Read the model definition and answer for the solid it produces. Units are mm, in the model's axes. Face numbers are marked on the shaded views. Coordinates: 2 decimals unless noted, no trailing zeros. Order: outer loops, then holes, each group sorted by start corner. A loop starts at its lowest first (then second) coordinate and runs counter-clockwise, first axis right, second up. Notation, with made-up numbers: (49, 62.25) - (104, 62.25) arc R23 cw to (104, 72.25) - close; hole circle Ø4 at (64, 36). An arc over 180 degrees is marked (long way). Write item = value, one per line.
from build123d import *

# Parameters (mm, degrees)
F1_DEPTH = 6.6802
F2_DEPTH = 3.2512
F4_DEPTH = 2.54


with BuildPart() as f1:
    # F0 (on Top) → F1 (new body)
    with BuildSketch(Plane.XY):
        Polygon((46.99, 18.161), (-46.99, 18.161), (-46.99, 4.401166), (-10.16, 4.401166), (10.16, 4.401166), (46.99, 4.401166), align=None)
    extrude(amount=F1_DEPTH)

    # F0 (on Top) → F2 (join)
    with BuildSketch(Plane.XY):
        with BuildLine():
            Line((-10.16, 4.401166), (-46.99, 4.401166))
            ThreePointArc((-46.99, 4.401166), (-40.386, -4.664891), (-46.99, -13.730948))
            Line((-46.99, -13.730948), (-46.99, -16.108993))
            ThreePointArc((-46.99, -16.108993), (-39.314297, -9.881174), (-39.060262, 0))
            Line((-39.060262, 0), (-10.16, 0))
            Line((-10.16, 0), (-10.16, 4.401166))
        make_face()
        with BuildLine():
            ThreePointArc((46.99, -13.730948), (40.386, -4.664891), (46.99, 4.401166))
            Line((46.99, 4.401166), (10.16, 4.401166))
            Line((10.16, 4.401166), (10.16, 0))
            Line((10.16, 0), (39.060262, 0))
            ThreePointArc((39.060262, 0), (39.314297, -9.881174), (46.99, -16.108993))
            Line((46.99, -16.108993), (46.99, -13.730948))
        make_face()
    extrude(amount=F2_DEPTH)

    # F3 (on face) → F4 (cut)
    with BuildSketch(Plane.XY):
        with BuildLine():
            Line((-46.99, 15.853083), (-46.99, 6.709083))
            ThreePointArc((-46.99, 6.709083), (-42.418, 11.281083), (-46.99, 15.853083))
        make_face()
        with BuildLine():
            ThreePointArc((46.99, 15.853083), (42.418, 11.281083), (46.99, 6.709083))
            Line((46.99, 6.709083), (46.99, 15.853083))
        make_face()
    extrude(amount=F4_DEPTH, mode=Mode.SUBTRACT)


solid = f1.part
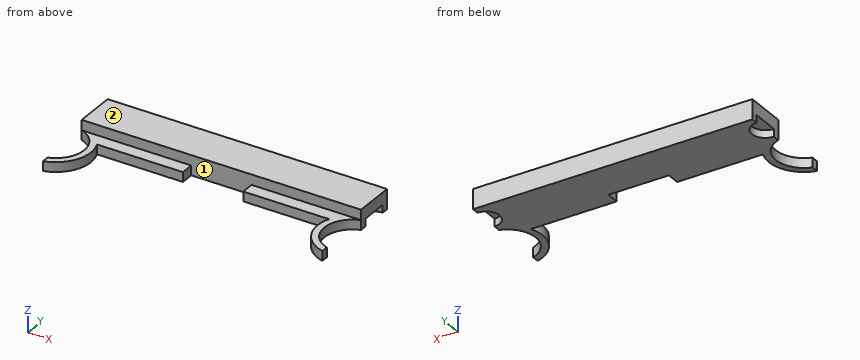
1) Determine the mould class of the marked faces 1 and 2 for opening direction X: pulls with the +X half, pulls with the -X half, needs draft (parallel to the pull), parting line crosses it, or undercut.
Returned:
face_1 = undercut
face_2 = needs draft
2) Flat-ended cylindrical pins translate along their axes: pin 1 Ø3.5 at (y, z) = (1.5, 1) entering from +X; pin 2 Ø3.5 at (x, z) = (-15.5, 2.5) entering from -Y; pin 3 Ø3.5 at (x, y) = (45, 9.5) entering from -Z; pin 4 Ø12 at (x, y) = (17, -8) entering from -Z. Find the tip coordinate at first contact, or state that the pin passes through.
Returned:
pin_1 = 44.61
pin_2 = 0
pin_3 = 2.54
pin_4 = through
3) The part is cut by section B-B (x = 26.5). Determine the outline of the cut face in (y, z), and give its area (3 significant figures).
Returned:
outline = (0, 0) - (18.16, 0) - (18.16, 6.68) - (4.4, 6.68) - (4.4, 3.25) - (0, 3.25) - close
area = 106 mm^2
4) The part is cut by section D-D (y = -10.5). Determine the outline of the cut face in (x, z).
Returned:
outline = (-42.38, 0) - (-39.64, 0) - (-39.64, 3.25) - (-42.38, 3.25) - close; (39.64, 0) - (42.38, 0) - (42.38, 3.25) - (39.64, 3.25) - close
5) Straight lines are drawn through the part: line 1 along Y through (x, z) = (-37, 2.5); line 2 along Y through (x, z) = (-13, 3.5); line 3 along X through (y, z) = (-12, 1.25). For each, find the intervals that lie inside material, in ascending order. Write a range as from..to.
Returned:
line_1 = 0..18.16
line_2 = 4.4..18.16
line_3 = -43.83..-40.65, 40.65..43.83
6) The part is cut by section A-A (y = 1). Determine the outline of the cut face in (x, z).
Returned:
outline = (-42.25, 0) - (-10.16, 0) - (-10.16, 3.25) - (-42.25, 3.25) - close; (10.16, 0) - (42.25, 0) - (42.25, 3.25) - (10.16, 3.25) - close
7) The part is cut by section C-C (y = 13). Determine the outline of the cut face in (x, z), and give its area (3 significant figures).
Returned:
outline = (-46.99, 2.54) - (-42.75, 2.54) - (-42.75, 0) - (42.75, 0) - (42.75, 2.54) - (46.99, 2.54) - (46.99, 6.68) - (-46.99, 6.68) - close
area = 606 mm^2
